Part model, mm, in its own coordinate system. Face numbers are marked on the shaded views. A direction names the side the tool comes from. Round coordinates to 2 decimals unless told otherwise and drop trailing zeros. Write each loop counter-clockwise with the first axis right and the second up, starting at its lowest first coordinate (ties: lowest second). Pieces come first, ordered by that corner, then holes. Notation, with made-up numbers: M 87,-20.5 L 94,-20.5 A27 ccw 94,3.5 Z; hole C 49,58 d1. An arc over 180 degrees is marked long. Answer as a JSON object with one key per item and string values. Group by question number.
1. Band-saw the part on B-B, the plane z = 14.5. Write the cut outline in (x, y), plus the area to 3 significant figures.
2. Band-saw the part on C-C, the plane y = 22.5. Write the cut outline in (x, z).
3. Which spindle directions (+Z, -Z, +X, -X, +Y, -Y) get a long thin tool onto all of the face, cutting with end or side? Do the marked faces 4 and 5. Say none if no direction does.
4. Band-saw the part on A-A, the plane x = 22.5. Write the cut outline in (y, z), plus the area to 3 significant figures.
5. Two-plate mould, pull along X, no slides. Class the marked faces 1, 2 and 3: +X half, -X half, draft (parallel to the pull), parting line (faces both ways), or undercut.
6. Drop flat-ended pins along their axis: pin 1 (2 mm diameter, centred on x = 58.5, y = 21, fed in from +Z); pin 2 (5 mm diameter, centred on x = -22.5, y = 22.5, fed in from +Z). Give the stop position or say it passes through.
7. Drill centre lines: line 1 (Y direction, x = 22.5, z = 7.75); line 2 (Y direction, x = 55, z = 14); line 3 (X direction, y = -5.5, z = 33). Where is each one in solid material? Low to high. Write a range as from..to.
8. Band-saw the part on D-D, the plane x = 0. Write the cut outline in (y, z).
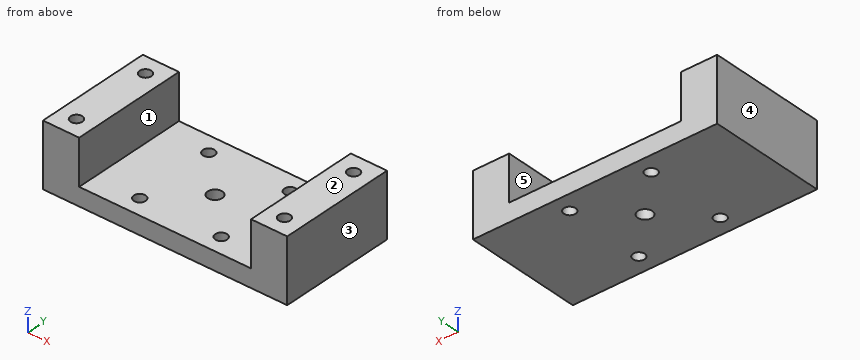
from build123d import *

# Parameters (mm, degrees)
F0_W     = 135
F0_H     = 65
F0_R     = 3.25
F0_R_2   = 4
F1_DEPTH = 10
F2_W     = 20
F2_H     = 65
F2_R     = 3.25
F3_DEPTH = 25


with BuildPart() as f1:
    # F0 (on Top) → F1 (new body)
    with BuildSketch(Plane.XY):
        Rectangle(F0_W, F0_H)
        with Locations((-22.5, -22.5)):
            Circle(F0_R, mode=Mode.SUBTRACT)
        with Locations((22.5, -22.5)):
            Circle(F0_R, mode=Mode.SUBTRACT)
        with Locations((-22.5, 22.5)):
            Circle(F0_R, mode=Mode.SUBTRACT)
        Circle(F0_R_2, mode=Mode.SUBTRACT)
        with Locations((22.5, 22.5)):
            Circle(F0_R, mode=Mode.SUBTRACT)
    extrude(amount=F1_DEPTH)

    # F2 (on face) → F3 (join)
    with BuildSketch(Plane.XY.offset(10)):
        with Locations((57.5, 0)):
            Rectangle(F2_W, F2_H)
        with Locations((57.5, -22.5)):
            Circle(F2_R, mode=Mode.SUBTRACT)
        with Locations((57.5, 22.5)):
            Circle(F2_R, mode=Mode.SUBTRACT)
        with Locations((-57.5, 0)):
            Rectangle(F2_W, F2_H)
        with Locations((-57.5, -22.5)):
            Circle(F2_R, mode=Mode.SUBTRACT)
        with Locations((-57.5, 22.5)):
            Circle(F2_R, mode=Mode.SUBTRACT)
    extrude(amount=F3_DEPTH)


solid = f1.part
Worked answers:
{
 "1": {"outline": "M -67.5,-32.5 L -47.5,-32.5 L -47.5,32.5 L -67.5,32.5 Z; M 47.5,-32.5 L 67.5,-32.5 L 67.5,32.5 L 47.5,32.5 Z; hole C -57.5,-22.5 d6.5; hole C -57.5,22.5 d6.5; hole C 57.5,-22.5 d6.5; hole C 57.5,22.5 d6.5", "area": "2,470 mm^2"},
 "2": {"outline": "M -67.5,0 L -25.75,0 L -25.75,10 L -47.5,10 L -47.5,35 L -54.25,35 L -54.25,10 L -60.75,10 L -60.75,35 L -67.5,35 Z; M -19.25,0 L 19.25,0 L 19.25,10 L -19.25,10 Z; M 25.75,0 L 67.5,0 L 67.5,35 L 60.75,35 L 60.75,10 L 54.25,10 L 54.25,35 L 47.5,35 L 47.5,10 L 25.75,10 Z"},
 "3": {"face 4": "+Z, -Z, -X, +Y, -Y", "face 5": "+Z, +Y, -Y"},
 "4": {"outline": "M -32.5,0 L -25.75,0 L -25.75,10 L -32.5,10 Z; M -19.25,0 L 19.25,0 L 19.25,10 L -19.25,10 Z; M 25.75,0 L 32.5,0 L 32.5,10 L 25.75,10 Z", "area": "520 mm^2"},
 "5": {"face 1": "undercut", "face 2": "draft", "face 3": "+X half"},
 "6": {"pin 1": "stops at z = 10", "pin 2": "passes through"},
 "7": {"line 1": "y = -32.5..-25.75, -19.25..19.25, 25.75..32.5", "line 2": "y = -32.5..-24.58, -20.42..20.42, 24.58..32.5", "line 3": "x = -67.5..-47.5, 47.5..67.5"},
 "8": {"outline": "M -32.5,0 L -4,0 L -4,10 L -32.5,10 Z; M 4,0 L 32.5,0 L 32.5,10 L 4,10 Z"}
}
